Check sheet for the modelled part. Datum: model origin and axes. Units: mm. Coordinates: 2 decimals unless noted, no trailing zeros. Write each loop counter-clockwise with the first axis right and the second up, starting at its lowest first coordinate (ties: lowest second). Pieces come first, ordered by that corner, then holes. Notation, with made-up numbers: (16, 2) - (67, 2) arc R10 cw to (67, 15) - close; hole circle Ø1 at (26.25, -5). An arc over 180 degrees is marked (long way). Write each question's results on one line, items separated by ' | '.
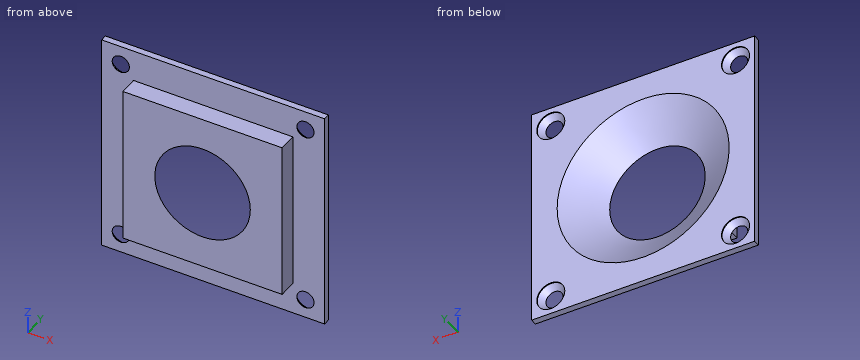
from build123d import *

# Parameters (mm, degrees)
SKETCH1_W                                      = 25
SKETCH1_H                                      = 25
BOSS_EXTRUDE1_DEPTH                            = 2.85
SKETCH2_W                                      = 35
SKETCH2_H                                      = 35
BOSS_EXTRUDE2_DEPTH                            = 1
CSK_FOR_M2_FLAT_HEAD_MACHINE_SCREW1_AT_2_COUNT = 2
CSK_FOR_M2_FLAT_HEAD_MACHINE_SCREW1_AT_2_PITCH = 29
CSK_FOR_M2_FLAT_HEAD_MACHINE_SCREW1_AT_3_COUNT = 2
CSK_FOR_M2_FLAT_HEAD_MACHINE_SCREW1_AT_3_PITCH = 41.012193309
CSK_FOR_M2_FLAT_HEAD_MACHINE_SCREW1_AT_4_COUNT = 2
CSK_FOR_M2_FLAT_HEAD_MACHINE_SCREW1_AT_4_PITCH = 29


with BuildPart() as part:
    # Sketch1 → Boss-Extrude1 (new body)
    with BuildSketch(Plane(origin=(0, 0, 0), x_dir=(1, 0, 0), z_dir=(0, 1, 0))):
        Rectangle(SKETCH1_W, SKETCH1_H)
    extrude(amount=BOSS_EXTRUDE1_DEPTH)

    # Sketch2 → Boss-Extrude2 (add)
    with BuildSketch(Plane(origin=(0, 2.85, 0), x_dir=(1, 0, 0), z_dir=(0, 1, 0))):
        Rectangle(SKETCH2_W, SKETCH2_H)
    extrude(amount=BOSS_EXTRUDE2_DEPTH)

    # Sketch3 → Cut-Revolve1 (revolve, cut)
    with BuildSketch(Plane.XY):
        Polygon((0, 0), (7.5, 0), (13.5, 3.85), (0, 3.85), align=None)
    revolve(axis=Axis((0, 0, 0), (0, 1, 0)), mode=Mode.SUBTRACT)

    # Sketch4 → CSK for M2 Flat Head Machine Screw1 (revolve, cut)
    with BuildSketch(Plane(origin=(-14.5, 3.85, -14.5), x_dir=(0, 0, 1), z_dir=(1, 0, 0))):
        Polygon((0, 0), (0, 10.721032743), (1.2, 10), (1.2, 1.15), (2.2, 0.15), (2.2, 0), align=None)
    csk_for_m2_flat_head_machine_screw1 = revolve(axis=Axis((-14.5, 10.2, -14.5), (0, -1, 0)), mode=Mode.SUBTRACT)

    # CSK for M2 Flat Head Machine Screw1 at 2: CSK for M2 Flat Head Machine Screw1 ×2
    with Locations(*[(i * CSK_FOR_M2_FLAT_HEAD_MACHINE_SCREW1_AT_2_PITCH, 0, 0) for i in range(1, CSK_FOR_M2_FLAT_HEAD_MACHINE_SCREW1_AT_2_COUNT)]):
        add(csk_for_m2_flat_head_machine_screw1, mode=Mode.SUBTRACT)

    # CSK for M2 Flat Head Machine Screw1 at 3: CSK for M2 Flat Head Machine Screw1 ×2
    with Locations(*[Vector(0.707106781, 0, 0.707106781) * (i * CSK_FOR_M2_FLAT_HEAD_MACHINE_SCREW1_AT_3_PITCH) for i in range(1, CSK_FOR_M2_FLAT_HEAD_MACHINE_SCREW1_AT_3_COUNT)]):
        add(csk_for_m2_flat_head_machine_screw1, mode=Mode.SUBTRACT)

    # CSK for M2 Flat Head Machine Screw1 at 4: CSK for M2 Flat Head Machine Screw1 ×2
    with Locations(*[(0, 0, i * CSK_FOR_M2_FLAT_HEAD_MACHINE_SCREW1_AT_4_PITCH) for i in range(1, CSK_FOR_M2_FLAT_HEAD_MACHINE_SCREW1_AT_4_COUNT)]):
        add(csk_for_m2_flat_head_machine_screw1, mode=Mode.SUBTRACT)


solid = part.part
1. Go/stop test with flat-tipped pins: pin 1 (3.5 mm diameter, centred on x = 14.5, z = 14.5, fed in from -Y); pin 2 (1.4 mm diameter, centred on x = 4, y = 1.5, fed in from +Z); pin 3 (2 mm diameter, centred on y = 1, z = -1.5, fed in from +X). Record where each tip stops, or that it passes through.
Values follow:
pin 1: stops at y = 2.85 | pin 2: stops at z = 12.5 | pin 3: stops at x = 12.5
2. Sectioned sample at C-C (z = 0). Record the cut outline in (x, y).
Values follow:
outline: (-17.5, 2.85) - (-12.5, 2.85) - (-12.5, 0) - (-7.5, 0) - (-13.5, 3.85) - (-17.5, 3.85) - close; (7.5, 0) - (12.5, 0) - (12.5, 2.85) - (17.5, 2.85) - (17.5, 3.85) - (13.5, 3.85) - close
3. Material ranges on L1, parallel to Z at x = 14.5, y = 3.8; L2, parallel to X at y = 3.4, z = 14, recorded low to high. Write a range as [from, to].
Values follow:
L1: z = [-17.5, -16.7], [-12.3, 12.3], [16.7, 17.5] | L2: x = [-17.5, -16.33], [-12.67, 12.67], [16.33, 17.5]
4. Sectioned sample at B-B (x = 0). Record the cut outline in (y, z).
Values follow:
outline: (0, -12.5) - (2.85, -12.5) - (2.85, -17.5) - (3.85, -17.5) - (3.85, -13.5) - (0, -7.5) - close; (0, 7.5) - (3.85, 13.5) - (3.85, 17.5) - (2.85, 17.5) - (2.85, 12.5) - (0, 12.5) - close
5. Sectioned sample at D-D (x = 14.5). Record the cut outline in (y, z), then the cut area to 3 significant figures.
Values follow:
outline: (2.85, -17.5) - (3.85, -17.5) - (3.85, -16.7) - (3.7, -16.7) - (2.85, -15.85) - close; (2.85, -13.15) - (3.7, -12.3) - (3.85, -12.3) - (3.85, 12.3) - (3.7, 12.3) - (2.85, 13.15) - close; (2.85, 15.85) - (3.7, 16.7) - (3.85, 16.7) - (3.85, 17.5) - (2.85, 17.5) - close | area: 27.6 mm^2
6. Sectioned sample at A-A (z = 14.5). Record the cut outline in (x, y).
Values follow:
outline: (-17.5, 2.85) - (-15.85, 2.85) - (-16.7, 3.7) - (-16.7, 3.85) - (-17.5, 3.85) - close; (-13.15, 2.85) - (13.15, 2.85) - (12.3, 3.7) - (12.3, 3.85) - (-12.3, 3.85) - (-12.3, 3.7) - close; (15.85, 2.85) - (17.5, 2.85) - (17.5, 3.85) - (16.7, 3.85) - (16.7, 3.7) - close
